Here's how the part is built. I have some questions about the finished solid (model axes, mm). A direction names the side the tool comes from. Give positions to 0.01 mm unless a question says otherwise; leave off trailing zeros. Write each loop counter-clockwise with the first axis right and the second up, starting at its lowest first coordinate (ties: lowest second). Pieces come first, ordered by that corner, then holes. Notation, with made-up numbers: (88.25, -34.75) -> (126.25, -34.75) arc R24 ccw to (126.25, -6.75) -> close; hole circle Ø2 at (40.5, 84). An arc over 180 degrees is marked (long way). Use CSV: the item, a comma, the result in double quotes. Start each with the question number.
(1) Which directions (+Z, -Z, +X, -X, +Y, -Y) give clear straight access to the entire face, cutting with the end or side of a thin tool? Please do faces 1 (the flat face through (2, -10.466, 57)), 2 (the flat face through (2, 16.534, 24)), 3 (the flat face through (2, 20.534, 22)).
(2) Suppose I cut it at B-B on x = 19. List the corners of the cut face in (y, z) for me.
(3) If we mould it in two halves opening along Z, with no side actions, what happens to faces 4 (the flat face through (2, -12, 55)), 5 (the flat face through (2, 1, 0)), 6 (the flat face through (2, -18.466, 29)), 7 (the flat face through (2, -14.466, 29))? For each: pulls with the +Z half, pulls with the -Z half, needs draft (parallel to the pull), parting line crosses it, or undercut.
(4) I need wall thicknesses on L1, parallel to Y at x = 19, z = 15; L2, parallel to Z at x = -15.5, y = -11.5; L3, parallel to Y at x = -2, z = 52. Which ranges of each line are inside material? Lowest first, please. Write a range as [from, to].
(5) Suppose I cut it at A-A on z = 24.5. List the corners of the cut face in (x, y) for me.
(6) Suppose I cut it at D-D on y = 18.5. List the corners of the cut face in (x, z) for me.
(7) Suppose I cut it at C-C on y = -3. List the corners of the cut face in (x, z) for me.
(8) For pin 1 Ø12 at (x, y) = (-10.5, -2) entering from +Z; pin 2 Ø1 at (x, z) = (-8.5, 57) entering from +Y; pin 3 Ø0.6 at (x, y) = (7.5, 18) entering from +Z, each with a flat end and sliding along its axis, tell me the tip position at first contact or that it passes through.
from build123d import *

# Parameters (mm, degrees)
ESBO_O1_W                = 45
ESBO_O1_H                = 35
RESSALTO_EXTRUS_O1_DEPTH = 4
ESBO_O2_W                = 45
ESBO_O2_H                = 45
RESSALTO_EXTRUS_O2_DEPTH = 4
ESBO_O3_W                = 45
ESBO_O3_H                = 4
RESSALTO_EXTRUS_O3_DEPTH = 55
ESBO_O4_W                = 45
ESBO_O4_H                = 4
RESSALTO_EXTRUS_O4_DEPTH = 4
FILETE1_R                = 1


with BuildPart() as part:
    # Esboço1 → Ressalto-extrusão1 (new body)
    with BuildSketch(Plane.XY):
        with Locations((2.182824508, -0.966135458)):
            Rectangle(ESBO_O1_W, ESBO_O1_H)
    extrude(amount=RESSALTO_EXTRUS_O1_DEPTH)

    # Esboço2 → Ressalto-extrusão2 (add)
    with BuildSketch(Plane(origin=(0, 16.533864542, 0), x_dir=(1, 0, 0), z_dir=(0, 1, 0))):
        with Locations((2.182824508, -22.5)):
            Rectangle(ESBO_O2_W, ESBO_O2_H)
    extrude(amount=RESSALTO_EXTRUS_O2_DEPTH)

    # Esboço3 → Ressalto-extrusão3 (add)
    with BuildSketch(Plane.XY.offset(4)):
        with Locations((2.182824508, -16.466135458)):
            Rectangle(ESBO_O3_W, ESBO_O3_H)
    extrude(amount=RESSALTO_EXTRUS_O3_DEPTH)

    # Esboço4 → Ressalto-extrusão4 (add)
    with BuildSketch(Plane(origin=(0, -14.466135458, 0), x_dir=(1, 0, 0), z_dir=(0, 1, 0))):
        with Locations((2.182824508, -57)):
            Rectangle(ESBO_O4_W, ESBO_O4_H)
    extrude(amount=RESSALTO_EXTRUS_O4_DEPTH)

    # Filete1
    filete1_edges = [part.edges().sort_by_distance(p)[0] for p in [
        (-20.317175492, 16.533864542, 24.5),
        (2.182824508, 16.533864542, 45),
        (-20.317175492, 18.533864542, 45),
        (24.682824508, 16.533864542, 24.5),
        (24.682824508, 18.533864542, 45),
        (2.182824508, 16.533864542, 4),
        (-20.317175492, 20.533864542, 22.5),
        (2.182824508, 20.533864542, 45),
        (24.682824508, 20.533864542, 22.5),
        (2.182824508, 20.533864542, 0),
        (24.682824508, 1.033864542, 4),
        (2.182824508, -14.466135458, 4),
        (24.682824508, -14.466135458, 59),
        (-20.317175492, -14.466135458, 59),
        (2.182824508, -18.466135458, 59),
        (-20.317175492, -14.466135458, 29.5),
        (24.682824508, -14.466135458, 29.5),
        (-20.317175492, -12.466135458, 55),
        (2.182824508, -14.466135458, 55),
        (24.682824508, -12.466135458, 55),
        (-20.317175492, -10.466135458, 57),
        (2.182824508, -10.466135458, 59),
        (24.682824508, -10.466135458, 57),
        (2.182824508, -10.466135458, 55),
        (-20.317175492, 1.033864542, 4),
        (24.682824508, 1.033864542, 0),
        (2.182824508, -18.466135458, 0),
        (-20.317175492, 1.033864542, 0),
        (24.682824508, -18.466135458, 29.5),
        (-20.317175492, -18.466135458, 29.5),
    ]]
    fillet(filete1_edges, radius=FILETE1_R)


solid = part.part
Geometry says:
1,face 1,"+Z, +X, -X, +Y"
1,face 2,"+Z, +X, -X"
1,face 3,"+Z, -Z, +X, -X, +Y"
2,outline,"(-18.47, 1) arc R1 ccw to (-17.47, 0) -> (19.53, 0) arc R1 ccw to (20.53, 1) -> (20.53, 44) arc R1 ccw to (19.53, 45) -> (17.53, 45) arc R1 ccw to (16.53, 44) -> (16.53, 5) arc R1 cw to (15.53, 4) -> (-13.47, 4) arc R1 cw to (-14.47, 5) -> (-14.47, 54) arc R1 cw to (-13.47, 55) -> (-11.47, 55) arc R1 ccw to (-10.47, 56) -> (-10.47, 58) arc R1 ccw to (-11.47, 59) -> (-17.47, 59) arc R1 ccw to (-18.47, 58) -> close"
3,face 4,"undercut"
3,face 5,"pulls with the -Z half"
3,face 6,"needs draft"
3,face 7,"undercut"
4,L1,"[-18.47, -14.47], [16.53, 20.53]"
4,L2,"[0, 4], [55, 59]"
4,L3,"[-18.47, -14.47]"
5,outline,"(-20.32, -17.47) arc R1 ccw to (-19.32, -18.47) -> (23.68, -18.47) arc R1 ccw to (24.68, -17.47) -> (24.68, -15.47) arc R1 ccw to (23.68, -14.47) -> (-19.32, -14.47) arc R1 ccw to (-20.32, -15.47) -> close; (-20.32, 17.53) arc R1 ccw to (-19.32, 16.53) -> (23.68, 16.53) arc R1 ccw to (24.68, 17.53) -> (24.68, 19.53) arc R1 ccw to (23.68, 20.53) -> (-19.32, 20.53) arc R1 ccw to (-20.32, 19.53) -> close"
6,outline,"(-20.32, 1) arc R1 ccw to (-19.32, 0) -> (23.68, 0) arc R1 ccw to (24.68, 1) -> (24.68, 44) arc R1 ccw to (23.68, 45) -> (-19.32, 45) arc R1 ccw to (-20.32, 44) -> close"
7,outline,"(-20.32, 1) arc R1 ccw to (-19.32, 0) -> (23.68, 0) arc R1 ccw to (24.68, 1) -> (24.68, 3) arc R1 ccw to (23.68, 4) -> (-19.32, 4) arc R1 ccw to (-20.32, 3) -> close"
8,pin 1,"z = 4"
8,pin 2,"y = -10.47"
8,pin 3,"z = 45"
